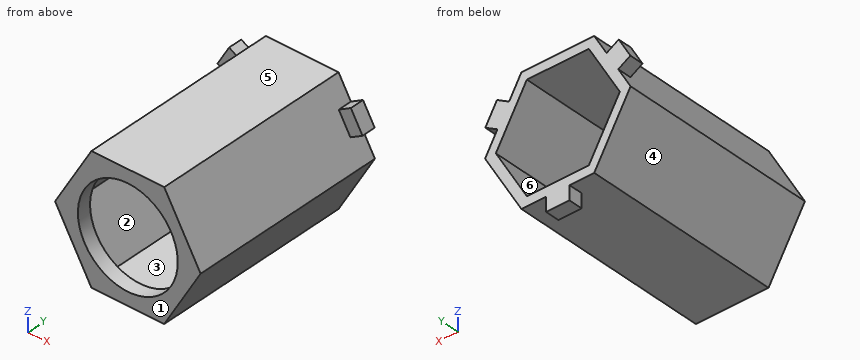
from build123d import *

# Parameters (mm, degrees)
SKETCH1_R           = 10.7
BOSS_EXTRUDE1_DEPTH = 43
CUT_EXTRUDE1_DEPTH  = 40
SKETCH3_W           = 5
SKETCH3_H           = 3
BOSS_EXTRUDE2_DEPTH = 3


with BuildPart() as part:
    # Sketch1 → Boss-Extrude1 (new body)
    with BuildSketch(Plane(origin=(0, 0, 0), x_dir=(1, 0, 0), z_dir=(0, 1, 0))):
        Polygon((15.588457268, 0), (7.794228634, 13.5), (-7.794228634, 13.5), (-15.588457268, 0), (-7.794228634, -13.5), (7.794228634, -13.5), align=None)
        with Locations(Location((0, 0, 0), (0, 0, 270))):
            Circle(SKETCH1_R, mode=Mode.SUBTRACT)
    extrude(amount=BOSS_EXTRUDE1_DEPTH)

    # Sketch2 → Cut-Extrude1 (cut)
    with BuildSketch(Plane(origin=(0, 43, 0), x_dir=(1, 0, 0), z_dir=(0, 1, 0))):
        Polygon((13.279056191, 0), (6.639528096, 11.5), (-6.639528096, 11.5), (-13.279056191, 0), (-6.639528096, -11.5), (6.639528096, -11.5), align=None)
    extrude(amount=-CUT_EXTRUDE1_DEPTH, mode=Mode.SUBTRACT)

    # Sketch3 → Boss-Extrude2 (add)
    with BuildSketch(Plane(origin=(0, 43, 0), x_dir=(1, 0, 0), z_dir=(0, 1, 0))):
        Polygon((15.539419162, -6.084936491), (12.941342951, -4.584936491), (10.441342951, -8.915063509), (13.039419162, -10.415063509), align=None)
        with Locations((0, 15)):
            Rectangle(SKETCH3_W, SKETCH3_H)
        Polygon((-13.039419162, -10.415063509), (-10.441342951, -8.915063509), (-12.941342951, -4.584936491), (-15.539419162, -6.084936491), align=None)
    extrude(amount=-BOSS_EXTRUDE2_DEPTH)


solid = part.part
Geometry: final body of the model. Coordinates: model frame, mm. Face numbers are marked on the shaded views. A direction names the side the tool comes from. Coordinates: 2 decimals unless noted, no trailing zeros. Order: outer loops, then holes, each group sorted by start corner. A loop starts at its lowest first (then second) coordinate and runs counter-clockwise, first axis right, second up.
(1) Draft query along Z for the marked faces 3, 4, 5 and 6. Return one class per face: pulls with the +Z half, pulls with the -Z half, needs draft (parallel to the pull), parting line crosses it, or undercut.
(2) Section query B-B (y = 24). Return the cut outline in (x, z), plus the area to 3 significant figures.
(3) Access query for the marked faces 1 and 2. Directions: +Z, -Z, +X, -X, +Y, -Y. A direction counts if a zero-diameter tool reaches every point of the face in a straight line with its end or side. Return the directions, or none.
(4) Section query D-D (x = -12). Return the cut outline in (y, z).
(5) Material intervals for probe 1 along Z at (x, y) = (-3, 19); probe 2 along X at (y, z) = (2.1, 0); probe 3 along Z at (x, y) = (0, 1), sorted ascending.
(6) First-contact query: pin 1 (1.5 mm diameter, centred on x = -12.5, z = 7.5, fed in from -Y); pin 2 (4 mm diameter, centred on x = 0.5, y = 21.5, fed in from -Z); pin 3 (2.5 mm diameter, centred on y = 41.5, z = -15.5, fed in from +X). Flat tips, straight axial feed; report the tip coordinate or a pass-through.
(7) Section query C-C (z = 7). Return the cut outline in (x, y).
(8) Section query A-A (x = 0). Return the cut outline in (y, z), plus the area to 3 significant figures.
Solution:
1. face 3: undercut
1. face 4: pulls with the -Z half
1. face 5: pulls with the +Z half
1. face 6: undercut
2. outline: (-15.59, 0) - (-7.79, -13.5) - (7.79, -13.5) - (15.59, 0) - (7.79, 13.5) - (-7.79, 13.5) - close; hole (-13.28, 0) - (-6.64, -11.5) - (6.64, -11.5) - (13.28, 0) - (6.64, 11.5) - (-6.64, 11.5) - close
2. area: 173 mm2
3. face 1: +Z, -Z, +X, -X, -Y
3. face 2: +Y
4. outline: (0, -6.22) - (43, -6.22) - (43, -2.22) - (3, -2.22) - (3, 2.22) - (43, 2.22) - (43, 9.81) - (40, 9.81) - (40, 6.22) - (0, 6.22) - close
5. probe 1: z = -13.5 to -11.5, 11.5 to 13.5
5. probe 2: x = -15.59 to -10.7, 10.7 to 15.59
5. probe 3: z = -13.5 to -10.7, 10.7 to 13.5
6. pin 1: stops at y = 40
6. pin 2: stops at z = -13.5
6. pin 3: stops at x = 2.5
7. outline: (-15.01, 40) - (-11.55, 40) - (-11.55, 0) - (-8.09, 0) - (-8.09, 3) - (-9.24, 3) - (-9.24, 43) - (-15.01, 43) - close; (8.09, 0) - (11.55, 0) - (11.55, 40) - (15.01, 40) - (15.01, 43) - (9.24, 43) - (9.24, 3) - (8.09, 3) - close
8. outline: (0, -13.5) - (40, -13.5) - (40, -16.5) - (43, -16.5) - (43, -11.5) - (3, -11.5) - (3, -10.7) - (0, -10.7) - close; (0, 10.7) - (3, 10.7) - (3, 11.5) - (43, 11.5) - (43, 13.5) - (0, 13.5) - close
8. area: 186 mm2
